Part print with two shaded views. Sizes in mm from the minimum x, y, z corner. A direction names the side the tool comes from. Coordinates: 2 decimals unless noted, no trailing zeros. Loops run counter-clockwise (first coordinate to the right, second up) from the corner with the lowest first, then second, coordinate; pieces in that order, holes last. Notation, with made-up numbers: (69, 72.25) -> (110, 72.25) arc R7 cw to (110, 78.25) -> close; hole circle Ø6 at (33.25, 77). An arc over 180 degrees is marked (long way). Answer as a JSON object with one key per item and string values. Group by question number.
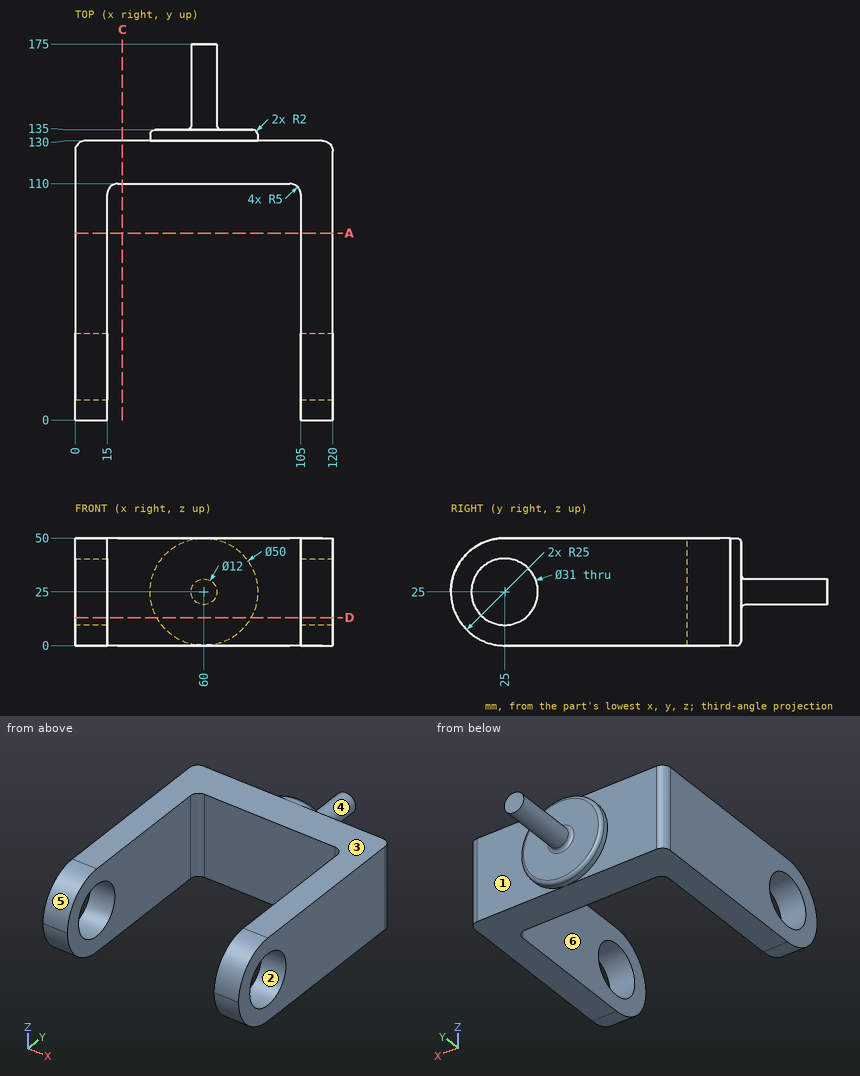
Item 1: Flat gauge pins, fed straight in: P1, Ø6, axis at x = 70.5, z = 7, coming from the +Y side; P2, Ø14, axis at x = 50, z = 15, coming from the +Y side. Where does each tip first touch, or does it go through?
Item 2: Band-saw the part on D-D, the plane z = 13. Count the separate pieces of the cut face and the enclosed holes in it, and give its area (3 significant figures).
Item 3: Band-saw the part on A-A, the plane y = 87. List the corners of the cut face in (x, z), and give its area (3 significant figures).
Item 4: Drill centre lines: L1, parallel to X at y = 29, z = 5; L2, parallel to Y at x = 77.5, z = 37; L3, parallel to X at y = 108, z = 37.5. Where is each one in solid material? Low to high.
Item 5: Pull direction Z, two halves, no side cores. Call the marked faces 1, 2 and 3: +Z half, -Z half, draft (parallel to the pull), parting line (faces both ways), or undercut.
Item 6: 3-axis set-ups, long thin cutter, end or side, ignore diameter. For the marked faces 4, 5 and 6: which of +Z, -Z, +X, -X, +Y, -Y reach the whole face in a straight line?
Item 7: Band-saw the part on C-C, the plane x = 22. List the corners of the cut face in (y, z).
Reply:
{
 "1": {"P1": "y = 135", "P2": "y = 135.19"},
 "2": {"separate pieces": "3", "enclosed holes": "0", "area": "5,240 mm²"},
 "3": {"outline": "(0, 0) -> (15, 0) -> (15, 50) -> (0, 50) -> close; (105, 0) -> (120, 0) -> (120, 50) -> (105, 50) -> close", "area": "1,500 mm²"},
 "4": {"L1": "0 to 15, 105 to 120", "L2": "110 to 135", "L3": "0 to 16, 104 to 120"},
 "5": {"face 1": "draft", "face 2": "undercut", "face 3": "+Z half"},
 "6": {"face 4": "+Y", "face 5": "+Z, +X, -X, -Y", "face 6": "+Z, -Z, -Y"},
 "7": {"outline": "(110, 0) -> (130, 0) -> (130, 50) -> (110, 50) -> close"}
}
